```python
from build123d import *

# Parameters (mm, degrees)
SKETCH1_W                                           = 55
SKETCH1_H                                           = 55
BOSS_EXTRUDE1_DEPTH                                 = 6
CBORE_FOR_M6_HEX_SOCKET_HEAD_CAP_SCREW1_D           = 6.6
CBORE_FOR_M6_HEX_SOCKET_HEAD_CAP_SCREW1_CBORE_D     = 11
CBORE_FOR_M6_HEX_SOCKET_HEAD_CAP_SCREW1_CBORE_DEPTH = 6.4
SKETCH4_W                                           = 55
SKETCH4_H                                           = 10
BOSS_EXTRUDE2_DEPTH                                 = 81
CBORE_FOR_M6_HEX_SOCKET_HEAD_CAP_SCREW2_D           = 6.6
CBORE_FOR_M6_HEX_SOCKET_HEAD_CAP_SCREW2_CBORE_D     = 11
CBORE_FOR_M6_HEX_SOCKET_HEAD_CAP_SCREW2_CBORE_DEPTH = 6.4
CHAMFER1_SIZE                                       = 70
CHAMFER1_SIZE2                                      = 25
F_6_0MM_DOWEL_HOLE1_D                               = 6


with BuildPart() as part:
    # Sketch1 → Boss-Extrude1 (new, symmetric)
    with BuildSketch(Plane.XY):
        Rectangle(SKETCH1_W, SKETCH1_H)
    extrude(amount=BOSS_EXTRUDE1_DEPTH, both=True)

    # CBORE for M6 Hex Socket Head Cap Screw1 (through all)
    with Locations(Plane.XY.offset(6)):
        with Locations((-20, 20), (20, 20), (20, -20), (-20, -20)):
            CounterBoreHole(CBORE_FOR_M6_HEX_SOCKET_HEAD_CAP_SCREW1_D / 2, CBORE_FOR_M6_HEX_SOCKET_HEAD_CAP_SCREW1_CBORE_D / 2, CBORE_FOR_M6_HEX_SOCKET_HEAD_CAP_SCREW1_CBORE_DEPTH)

    # Sketch4 → Boss-Extrude2 (add)
    with BuildSketch(Plane.XY.offset(6)):
        with Locations((0, -8)):
            Rectangle(SKETCH4_W, SKETCH4_H)
    extrude(amount=BOSS_EXTRUDE2_DEPTH)

    # CBORE for M6 Hex Socket Head Cap Screw2 (through all)
    with Locations(Plane(origin=(0, -13, 0), x_dir=(-1, 0, 0), z_dir=(0, -1, 0))):
        with Locations((-17.5, -76), (-7.5, -56), (-17.5, -36)):
            CounterBoreHole(CBORE_FOR_M6_HEX_SOCKET_HEAD_CAP_SCREW2_D / 2, CBORE_FOR_M6_HEX_SOCKET_HEAD_CAP_SCREW2_CBORE_D / 2, CBORE_FOR_M6_HEX_SOCKET_HEAD_CAP_SCREW2_CBORE_DEPTH)

    # Chamfer1
    chamfer1_edges = [part.edges().sort_by_distance(p)[0] for p in [
        (-27.5, -8, 87),
    ]]
    chamfer1_side = [part.faces().sort_by_distance(p)[0] for p in [
        (-27.5, -4.408163265, 25.62244898),
    ]]
    chamfer(chamfer1_edges, length=CHAMFER1_SIZE, length2=CHAMFER1_SIZE2, reference=chamfer1_side[0])

    # Ø6.0mm Dowel Hole1 (through all)
    with Locations(Plane(origin=(0, -13, 0), x_dir=(-1, 0, 0), z_dir=(0, -1, 0))):
        with Locations((-7.5, -36), (-7.5, -76)):
            Hole(F_6_0MM_DOWEL_HOLE1_D / 2)


solid = part.part
```
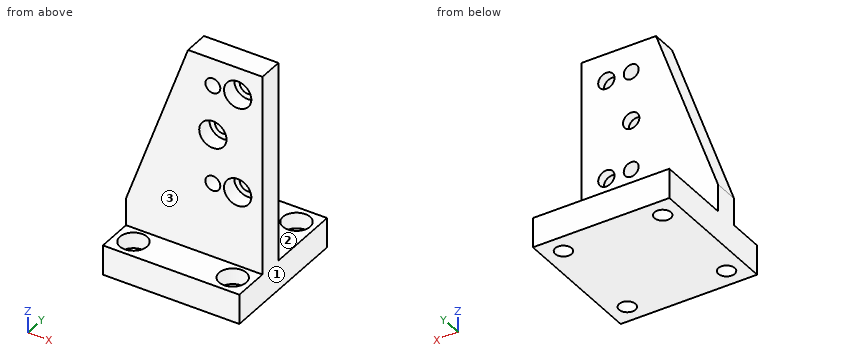
Verification items for the finished model (mm, model axes). Face numbers are marked on the shaded views. A direction names the side the tool comes from. Give positions to 0.01 mm unless a question says otherwise; leave off trailing zeros. Write each loop counter-clockwise with the first axis right and the second up, starting at its lowest first coordinate (ties: lowest second). Pieces come first, ordered by that corner, then holes. Notation, with made-up numbers: M 30,-31.5 L 60,-31.5 A21 ccw 60,2.5 Z; hole C -15,-16.75 d9. An arc over 180 degrees is marked long. One line per question, with ' | ' between items.
1) Gauge pin test, flat ends, axial feed: pin 1 Ø9 at (x, y) = (4, 20) entering from +Z; pin 2 Ø14.5 at (x, z) = (7.5, 56) entering from -Y; pin 3 Ø10.5 at (x, y) = (-20, -20) entering from +Z. Record the tip position at first contact, or that the pin passes through.
Result:
pin 1: stops at z = 6 | pin 2: stops at y = -13 | pin 3: stops at z = -0.4
2) Section check A-A on z = 4.5. Enter the section's corners in (x, y).
Result:
outline: M -27.5,-27.5 L 27.5,-27.5 L 27.5,27.5 L -27.5,27.5 Z; hole C -20,-20 d11; hole C -20,20 d11; hole C 20,-20 d11; hole C 20,20 d11
3) Section check B-B on x = 7.5. Enter the section's corners in (y, z), plus the area to 3 significant figures.
Result:
outline: M -27.5,-6 L 27.5,-6 L 27.5,6 L -3,6 L -3,33 L -13,33 L -13,6 L -27.5,6 Z; M -13,39 L -3,39 L -3,52.7 L -6.6,52.7 L -6.6,50.5 L -13,50.5 Z; M -13,61.5 L -6.6,61.5 L -6.6,59.3 L -3,59.3 L -3,73 L -13,73 Z; M -13,79 L -3,79 L -3,87 L -13,87 Z | area: 1,260 mm2
4) Section check D-D on x = 1. Enter the section's corners in (y, z).
Result:
outline: M -27.5,-6 L 27.5,-6 L 27.5,6 L -3,6 L -3,87 L -13,87 L -13,6 L -27.5,6 Z
5) Thickness scan on line 1 along Z through (x, y) = (17, -5); line 2 along Y through (x, z) = (17, 24); line 3 along X through (y, z) = (-10, 36). Record the ranges inside material, lowest first. Write a range as [from, to].
Result:
line 1: z = [-6, 32.74], [39.26, 72.74], [79.26, 87] | line 2: y = [-13, -3] | line 3: x = [-20.71, 4.5], [10.5, 12], [23, 27.5]
6) Section check C-C on y = -20. Enter the section's corners in (x, z).
Result:
outline: M -27.5,-6 L -23.3,-6 L -23.3,-0.4 L -25.5,-0.4 L -25.5,6 L -27.5,6 Z; M -16.7,-6 L 16.7,-6 L 16.7,-0.4 L 14.5,-0.4 L 14.5,6 L -14.5,6 L -14.5,-0.4 L -16.7,-0.4 Z; M 23.3,-6 L 27.5,-6 L 27.5,6 L 25.5,6 L 25.5,-0.4 L 23.3,-0.4 Z
7) Set-up check for the marked faces 1, 2 and 3: record each of +Z, -Z, +X, -X, +Y, -Y from which the full face is reachable in a straight line by a thin tool's end or side.
Result:
face 1: +Z, -Z, +X, +Y, -Y | face 2: +Z, +X, -X, +Y | face 3: +Z, +X, -X, -Y
